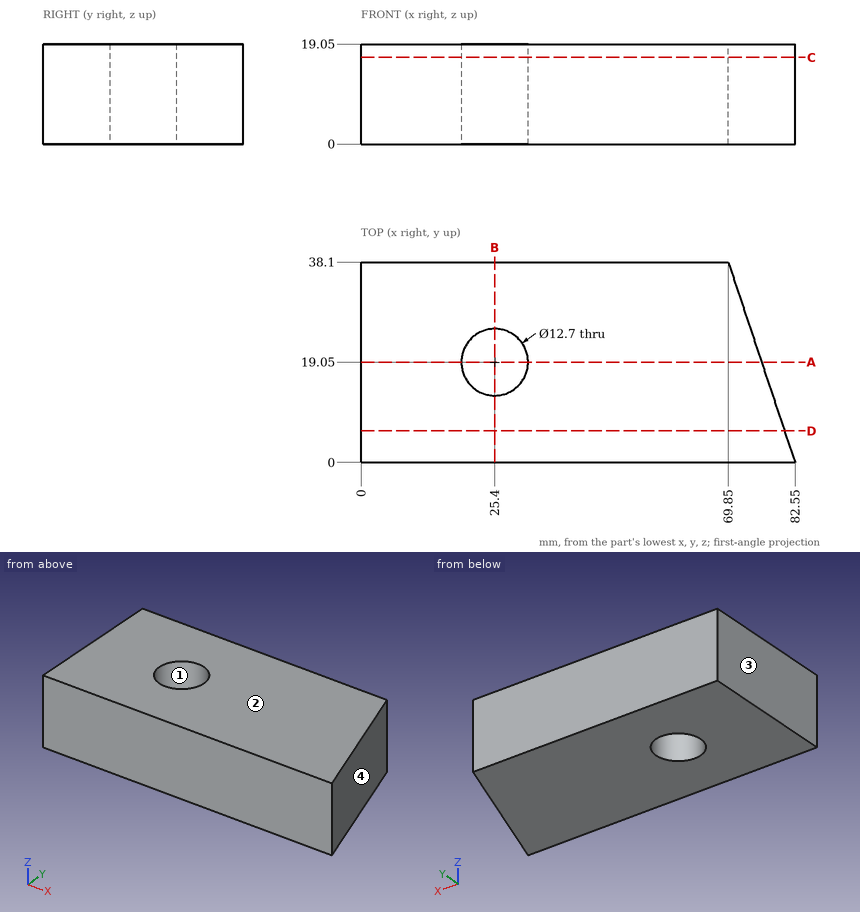
Drawing for the job (mm, zero at the part's lowest x, y, z). Round coordinates to 2 decimals unless told otherwise and drop trailing zeros. Loops run counter-clockwise (first coordinate to the right, second up) from the corner with the lowest first, then second, coordinate; pieces in that order, holes last. Notation, with made-up numbers: (64, -9.75) -> (84, -9.75) arc R18 cw to (84, 16.25) -> close; hole circle Ø9 at (13.5, -39). An arc over 180 degrees is marked (long way). Use one line per item in the form item = value. Start each with the question number.
Item 1: Band-saw the part on A-A (y = 19.05). List the corners of the cut face in (x, z), plus the area to 3 significant figures.
Item 2: Band-saw the part on B-B (x = 25.4). List the corners of the cut face in (y, z).
Item 3: Band-saw the part on C-C (z = 16.5). List the corners of the cut face in (x, y), plus the area to 3 significant figures.
Item 4: Drop flat-ended pins along their axis: pin 1 Ø6 at (y, z) = (4.5, 8) entering from +X; pin 2 Ø16.5 at (x, y) = (25.4, 19.05) entering from -Z; pin 3 Ø5 at (y, z) = (18.5, 16) entering from +X. Give the stop position or say it passes through.
Item 5: Drill centre lines: line 1 along Y through (x, z) = (25.4, 13.5); line 2 along X through (y, z) = (22, 8.25); line 3 along X through (y, z) = (23, 8.5). Where is each one in solid material? Low to high.
Item 6: Band-saw the part on D-D (y = 6). List the corners of the cut face in (x, z), plus the area to 3 significant figures.
Item 7: Two-plate mould, pull along X, no slides. Class the marked faces 1, 2, 3 and 4: released by +X, released by -X, zero draft, split by the parting line, or undercut.
Data:
q1.outline = (0, 0) -> (19.05, 0) -> (19.05, 19.05) -> (0, 19.05) -> close; (31.75, 0) -> (76.2, 0) -> (76.2, 19.05) -> (31.75, 19.05) -> close
q1.area = 1,210 mm^2
q2.outline = (0, 0) -> (12.7, 0) -> (12.7, 19.05) -> (0, 19.05) -> close; (25.4, 0) -> (38.1, 0) -> (38.1, 19.05) -> (25.4, 19.05) -> close
q3.outline = (0, 0) -> (82.55, 0) -> (69.85, 38.1) -> (0, 38.1) -> close; hole circle Ø12.7 at (25.4, 19.05)
q3.area = 2,780 mm^2
q4.pin_1 = 82.05
q4.pin_2 = 0
q4.pin_3 = 77.22
q5.line_1 = 0 to 12.7, 25.4 to 38.1
q5.line_2 = 0 to 19.78, 31.02 to 75.22
q5.line_3 = 0 to 20.43, 30.37 to 74.88
q6.outline = (0, 0) -> (80.55, 0) -> (80.55, 19.05) -> (0, 19.05) -> close
q6.area = 1,530 mm^2
q7.face_1 = undercut
q7.face_2 = zero draft
q7.face_3 = released by -X
q7.face_4 = released by +X
